Autodesk Inventor part; units mm, degrees
ref_plane "YZ Plane" through (0, 0, 0) normal (1, 0, 0) x (0, 1, 0)
ref_plane "XZ Plane" through (0, 0, 0) normal (0, 1, 0) x (-1, 0, 0)
ref_plane "XY Plane" through (0, 0, 0) normal (0, 0, 1) x (1, 0, 0)
sketch "Sketch1" plane through (0, 0, 0) normal (0, 1, 0) x (-1, 0, 0)
  arc A0 (0, -25.4) -> (0, 25.4) centre (0, 0) ccw
  arc A1 (-50.8, 25.4) -> (-50.8, -25.4) centre (-50.8, 0) ccw
  line L0 (0, 25.4) -> (-50.8, 25.4)
  line L1 (0, -25.4) -> (-50.8, -25.4)
  dimension "d0" = 50.8
extrude "Extrusion1" add sketch "Sketch1" along normal blind 6.35
sketch "Sketch2" plane through (0, 6.35, 0) normal (0, 1, 0) x (1, 0, 0)
  arc A0 (0, 19.05) -> (0, -19.05) centre (0, 0) ccw
  line L0 (0, 19.05) -> (38.1, 19.05)
  line L1 (0, -19.05) -> (38.1, -19.05)
  arc A1 (50.8, -25.4) -> (50.8, 25.4) centre (50.8, 0) ccw
  arc A2 (64.999, -12.7) -> (64.999, 12.7) centre (50.8, 0) ccw
  line L2 (50.8, 12.7) -> (64.999, 12.7)
  line L3 (50.8, -12.7) -> (64.999, -12.7)
  line L4 (50.8, -12.7) -> (38.1, -12.7)
  line L5 (50.8, 12.7) -> (38.1, 12.7)
  line L6 (38.1, 19.05) -> (38.1, 12.7)
  line L7 (38.1, -19.05) -> (38.1, -12.7)
  dimension "d6" = 38.1
  dimension "d7" = 38.1
extrude "Extrusion2" add sketch "Sketch2" along normal blind 12.7
sketch "Sketch3" plane through (0, 19.05, 0) normal (0, 1, 0) x (1, 0, 0)
  circle A0 centre (0, 0) radius 12.7
  dimension "d13" = 25.4
extrude "Extrusion3" cut sketch "Sketch3" against normal blind 25.4
sketch "Sketch4" plane through (0, 19.05, 0) normal (0, 1, 0) x (1, 0, 0)
  arc A0 (64.999, -12.7) -> (64.999, 12.7) centre (50.8, 0) ccw
  circle A1 centre (50.8, 0) radius 6.35
  point P0 (0, 0)
  dimension "d16" = 12.7
extrude "Extrusion4" add sketch "Sketch4" along normal blind 6.35
Could you check a few things on this model? Use its own coordinates, in mm. A direction names the side the tool comes from. Round coordinates to 2 decimals unless told otherwise and drop trailing zeros. Order: outer loops, then holes, each group sorted by start corner. A loop starts at its lowest first (then second) coordinate and runs counter-clockwise, first axis right, second up.
Q1. Please list where these lines run through material, in increasing order: probe 1 along X at (y, z) = (14.75, 0.5); probe 2 along Z at (x, y) = (0, 8); probe 3 along X at (y, z) = (5.75, 0).
Geometry says:
probe 1: x = -19.04 to -12.69, 12.69 to 69.84
probe 2: z = -19.05 to -12.7, 12.7 to 19.05
probe 3: x = -25.4 to -12.7, 12.7 to 76.2
Q2. Imagine slicing it at B-B, the plane z = 10. List the corners of the cut face in (x, y) for me, then the cut area to 3 significant figures.
Geometry says:
outline: (-23.35, 0) - (-7.83, 0) - (-7.83, 19.05) - (-16.21, 19.05) - (-16.21, 6.35) - (-23.35, 6.35) - close; (7.83, 0) - (74.15, 0) - (74.15, 6.35) - (67.01, 6.35) - (67.01, 19.05) - (7.83, 19.05) - close
area: 1,380 mm2
Q3. Imagine slicing it at D-D, the plane x = 19.5. List the corners of the cut face in (y, z) for me.
Geometry says:
outline: (0, -25.4) - (6.35, -25.4) - (6.35, -19.05) - (19.05, -19.05) - (19.05, 19.05) - (6.35, 19.05) - (6.35, 25.4) - (0, 25.4) - close
Q4. I'm going to push flat-ended pins straight in: P1, Ø4, axis at x = 13.5, y = 13, coming from the -Z side; P2, Ø4, axis at x = 24.5, z = -2.5, coming from the +Y side; P3, Ø2, axis at x = 59, y = 15, coming from the -Z side. Where does each tip first touch, or does it pass through?
Geometry says:
P1: stops at z = -19.05
P2: stops at y = 19.05
P3: stops at z = -12.7
Q5. Thinking about a two-plate mould opening in X: for faces 1 (the face through (25, 19.05, 0)), 2 (the face through (-2.75, 9.66, 12.4)), 3 (the face through (-19.045, 12.611, 0.419)), which applies, released by +X, released by -X, zero draft, split by the parting line, or undercut?
Geometry says:
face 1: zero draft
face 2: undercut
face 3: released by -X
Q6. Imagine slicing it at A-A, the plane y = 8.75. List the corners of the cut face in (x, z) for me, then the cut area to 3 significant figures.
Geometry says:
outline: (0, -19.05) - (38.1, -19.05) - (38.1, -12.7) - (65, -12.7) arc R19.05 ccw to (65, 12.7) - (38.1, 12.7) - (38.1, 19.05) - (0, 19.05) arc R19.05 ccw to start; hole circle Ø25.4 at (0, 0)
area: 2,280 mm2
Q7. Imagine slicing it at C-C, the plane x = 4. List the corners of the cut face in (y, z) for me, then the cut area to 3 significant figures.
Geometry says:
outline: (0, -25.4) - (6.35, -25.4) - (6.35, -19.05) - (19.05, -19.05) - (19.05, -12.05) - (0, -12.05) - close; (0, 12.05) - (19.05, 12.05) - (19.05, 19.05) - (6.35, 19.05) - (6.35, 25.4) - (0, 25.4) - close
area: 347 mm2
Q8. Which directions (+Z, -Z, +X, -X, +Y, -Y) give clear straight access to the entire face, cutting with the end or side of a thin tool? Please do faces 4 (the face through (38.1, 13, -16)), 5 (the face through (19, 13, 19.05)), 6 (the face through (69.85, 12.61, -0.19)), 7 (the face through (56.857, 22.181, 1.907)).
Geometry says:
face 4: -Z, +X, +Y
face 5: +Z, +X, -X, +Y
face 6: +X, +Y
face 7: +Y
